Could you check a few things on this model? Use its own coordinates, in mm. A direction names the side the tool comes from. Give positions to 0.01 mm unless a question says otherwise; leave off trailing zeros. Order: outer loops, then holes, each group sorted by start corner. A loop starts at its lowest first (then second) coordinate and runs counter-clockwise, first axis right, second up. Notation, with made-up numbers: M 9,-27.5 L 51,-27.5 A9 ccw 51,-13.5 Z; hole C -21,15 d4. An arc over 180 degrees is marked long. Use a Markdown table: item, result. Add a question column.
Item 1: If we mould it in two halves opening along X, with no side actions, what happens to faces 4 (the face through (-13.1, -22.14, 1.52)), 5 (the face through (0, 23, 1)), 6 (the face through (-7.9, 16.9, 1.5))? For each: released by +X, released by -X, zero draft, split by the parting line, or undercut.
Item 2: Suppose I cut it at C-C on z = 0.5. Write out the boundary of the cut face in (x, y), plus the area to 3 significant figures.
Item 3: Suppose I cut it at D-D on y = 4.5. Write out the boundary of the cut face in (x, z).
Item 4: Suppose I cut it at A-A on y = -18. Write out the boundary of the cut face in (x, z), plus the area to 3 significant figures.
Item 5: I'm going to push flat-ended pins straight in: pin 1 Ø2.5 at (x, y) = (-9, 18) entering from -Z; pin 2 Ø6 at (x, y) = (-5, -3) entering from -Z. Where does each tip first touch, or does it pass through?
Item 6: If I drill on L1, parallel to Y at x = -9, z = 2.2; L2, parallel to Y at x = 9, z = 1; L3, parallel to Y at x = 1, z = 2.9, over which ranges is the centre line in solid material (lowest first)? Write a range as from..to.
Item 7: Suppose I cut it at B-B on x = 9. Write out the boundary of the cut face in (y, z), plus the area to 3 significant figures.
Item 8: For faces 1 (the face through (10, 0, 1)), 2 (the face through (0, -23, 1)), 3 (the face through (0, 7, 2)), which set-ups out of +Z, -Z, +X, -X, +Y, -Y let a thin tool reach every point of the face, with its end or its side?
from build123d import *

# Parameters (mm, degrees)
SKETCH2_W                  = 46
SKETCH2_H                  = 28
SKETCH2_W_2                = 14
SKETCH2_H_2                = 14
BOSS_EXTRUDE1_DEPTH        = 3
F_2_6_2_6_DIAMETER_HOLE1_D = 2.6
SKETCH2_6_R                = 2.5
SKETCH2_6_W                = 20
SKETCH2_6_H                = 20
CUT_EXTRUDE2_DEPTH         = 1.5
FILLET1_R                  = 3


with BuildPart() as part:
    # Sketch2 → Boss-Extrude1 (new body)
    with BuildSketch(Plane(origin=(0, 0, 0), x_dir=(0, 1, 0), z_dir=(0, 0, 1))):
        Rectangle(SKETCH2_W, SKETCH2_H)
        Rectangle(SKETCH2_W_2, SKETCH2_H_2, mode=Mode.SUBTRACT)
    extrude(amount=BOSS_EXTRUDE1_DEPTH)

    # 2.6 _2.6_ Diameter Hole1 (through all)
    with Locations(Plane(origin=(0, 0, 0), x_dir=(-1, 0, 0), z_dir=(0, 0, -1))):
        with Locations((-9, -18), (9, -18), (-9, 18), (9, 18)):
            Hole(F_2_6_2_6_DIAMETER_HOLE1_D / 2)

    # Sketch2_6 → Cut-Extrude2 (cut)
    with BuildSketch(Plane(origin=(0, 0, 0), x_dir=(0, 1, 0), z_dir=(0, 0, 1))):
        with Locations(Location((-18, -9, 0), (0, 0, 270))):
            Circle(SKETCH2_6_R)
        with Locations(Location((-18, 9, 0), (0, 0, 270))):
            Circle(SKETCH2_6_R)
        with Locations(Location((18, 9, 0), (0, 0, 270))):
            Circle(SKETCH2_6_R)
        with Locations(Location((18, -9, 0), (0, 0, 270))):
            Circle(SKETCH2_6_R)
        Rectangle(SKETCH2_6_W, SKETCH2_6_H)
    extrude(amount=CUT_EXTRUDE2_DEPTH, mode=Mode.SUBTRACT)

    # Fillet1
    fillet1_edges = [part.edges().sort_by_distance(p)[0] for p in [
        (-14, 23, 1.5),
        (14, 23, 1.5),
        (14, -23, 1.5),
        (-14, -23, 1.5),
    ]]
    fillet(fillet1_edges, radius=FILLET1_R)


solid = part.part
Findings below:
| question | item | result |
|---|---|---|
| 1 | face 4 | released by -X |
| 1 | face 5 | zero draft |
| 1 | face 6 | undercut |
| 2 | outline | M -14,-20 A3 ccw -11,-23 L 11,-23 A3 ccw 14,-20 L 14,20 A3 ccw 11,23 L -11,23 A3 ccw -14,20 Z; hole C -9,-18 d5; hole C -9,18 d5; hole M -10,-10 L 10,-10 L 10,10 L -10,10 Z; hole C 9,-18 d5; hole C 9,18 d5 |
| 2 | area | 802 mm^2 |
| 3 | outline | M -14,0 L -10,0 L -10,1.5 L -7,1.5 L -7,3 L -14,3 Z; M 7,1.5 L 10,1.5 L 10,0 L 14,0 L 14,3 L 7,3 Z |
| 4 | outline | M -14,0 L -11.5,0 L -11.5,1.5 L -10.3,1.5 L -10.3,3 L -14,3 Z; M -7.7,1.5 L -6.5,1.5 L -6.5,0 L 6.5,0 L 6.5,1.5 L 7.7,1.5 L 7.7,3 L -7.7,3 Z; M 10.3,1.5 L 11.5,1.5 L 11.5,0 L 14,0 L 14,3 L 10.3,3 Z |
| 4 | area | 61.2 mm^2 |
| 5 | pin 1 | passes through |
| 5 | pin 2 | stops at z = 1.5 |
| 6 | L1 | y = -23..-19.3, -16.7..16.7, 19.3..23 |
| 6 | L2 | y = -23..-20.5, -15.5..-10, 10..15.5, 20.5..23 |
| 6 | L3 | y = -23..-7, 7..23 |
| 7 | outline | M -23,0 L -20.5,0 L -20.5,1.5 L -19.3,1.5 L -19.3,3 L -23,3 Z; M -16.7,1.5 L -15.5,1.5 L -15.5,0 L -10,0 L -10,1.5 L 10,1.5 L 10,0 L 15.5,0 L 15.5,1.5 L 16.7,1.5 L 16.7,3 L -16.7,3 Z; M 19.3,1.5 L 20.5,1.5 L 20.5,0 L 23,0 L 23,3 L 19.3,3 Z |
| 7 | area | 85.2 mm^2 |
| 8 | face 1 | -Z |
| 8 | face 2 | +Z, -Z, +X, -X, -Y |
| 8 | face 3 | +Z, -Z |
